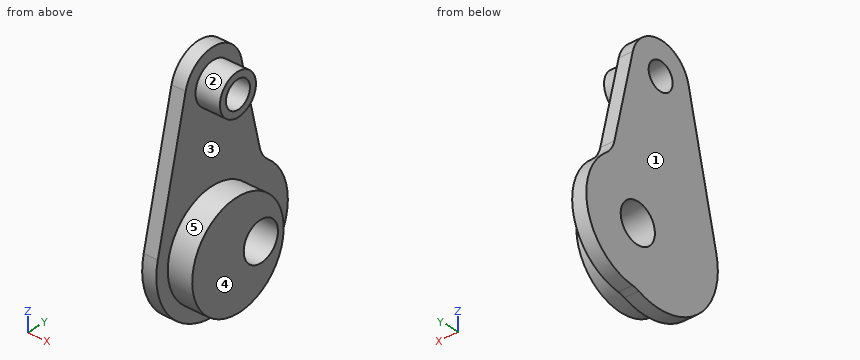
Autodesk Inventor part; units mm, degrees
ref_plane "YZ Plane" through (0, 0, 0) normal (1, 0, 0) x (0, 1, 0)
ref_plane "XZ Plane" through (0, 0, 0) normal (0, 1, 0) x (-1, 0, 0)
ref_plane "XY Plane" through (0, 0, 0) normal (0, 0, 1) x (1, 0, 0)
sketch "スケッチ1" plane through (0, 0, 0) normal (1, 0, 0) x (0, 1, 0)
  line L0 (0, 0) -> (0, -11) construction
  arc A0 (2.4346, 0.5682) -> (-2.4346, 0.5682) centre (0, 0) ccw
  circle A1 centre (0, -11) radius 4 construction
  line L1 (-2.4346, 0.5682) -> (-4.8692, -9.8636)
  arc A2 (0, -2.5) -> (2.4346, 0.5682) centre (0, 0) ccw construction
  arc A3 (-2.4346, 0.5682) -> (0, -2.5) centre (0, 0) ccw construction
  arc A4 (-4.8692, -9.8636) -> (1.9196, -15.6168) centre (0, -11) ccw
  arc A5 (-0.8211, -15.9321) -> (2.1875, -15.4961) centre (0, -11) ccw construction
  line L2 (2.4346, 0.5682) -> (4.043, -6.3238)
  arc A6 (2.476, -15.4748) -> (4.7628, -7.448) centre (2, -11) ccw
  line L3 (0, -11) -> (2, -11) construction
  arc A7 (0, -6) -> (-4.8692, -9.8636) centre (0, -11) ccw construction
  arc A8 (4.043, -6.3238) -> (4.7628, -7.448) centre (5.9907, -5.8693) ccw
  arc A9 (2.476, -15.4748) -> (1.9196, -15.6168) centre (2.6875, -17.4635) ccw
  point P0 (4.221, -7.0863)
  dimension "d1" = 11
  dimension "d2" = 8
  dimension "d4" = 2.5
  dimension "d39" = 5
  dimension "d54" = 2
  dimension "d55" = 4.5
  dimension "d56" = 2
extrude "押し出し1" add sketch "スケッチ1" along normal blind 1.1
sketch "スケッチ2" plane through (1.1, 0, 0) normal (1, 0, 0) x (0, 0, -1)
  circle A0 centre (0, 0) radius 1.575
  circle A1 centre (11, 0) radius 4
  line L0 (0, 0) -> (11, 0) construction
  arc A2 (9.8636, -4.8692) -> (15.6168, 1.9196) centre (11, 0) ccw construction
  point P0 (8.75, 4.8412)
  dimension "d12" = 3.15
  dimension "d13" = 8
extrude "押し出し2" add sketch "スケッチ2" along normal blind 1.9
sketch "スケッチ3" plane through (1.1, 0, 0) normal (1, 0, 0) x (0, 0, -1)
  point P0 (0, 0)
sketch "スケッチ4" plane through (0, 0, 0) normal (-1, 0, 0) x (0, 0, 1)
  arc A0 (0.5682, -2.4346) -> (0.5682, 2.4346) centre (0, 0) ccw construction
  arc A1 (-15.6168, 1.9196) -> (-9.8636, -4.8692) centre (-11, 0) ccw construction
  line L0 (-11, 0) -> (-11, 2) construction
  dimension "d53" = 2
hole "穴3" at (0, 0, 0) direction (1, 0, 0) diameter 2.1 end through all
hole "穴4" at (0, 2, -11) direction (1, 0, 0) diameter 2.99 end through all
properties part number "UPPER_LEG_BELT_TENSIONER"
Could you check a few things on this model? Use its own coordinates, in mm. Face numbers are marked on the shaded views. A direction names the side the tool comes from. Coordinates: 2 decimals unless noted, no trailing zeros. Order: outer loops, then holes, each group sorted by start corner. A loop starts at its lowest first (then second) coordinate and runs counter-clockwise, first axis right, second up. Notation, with made-up numbers: (-8.5, 35.5) -> (28.5, 35.5) arc R23 ccw to (28.5, 55.5) -> close; hole circle Ø5 at (78, -14.75). An arc over 180 degrees is marked (long way). One line per item, written item: value. Start each with the question number.
1) Imagine slicing it at D-D on x = 0.55. List the corners of the cut face in (y, z) for me (3 decimals), plus the area to 3 significant figures.
2) We'd pull the mould along Z, two halves only. Please class the marked faces 1, 2 and 3: +Z half, -Z half, draft (parallel to the pull), parting line (faces both ways), or undercut.
3) Imagine slicing it at C-C on x = 1.7. List the corners of the cut face in (y, z) for me (3 decimals).
4) Imagine slicing it at B-B on y = 0. List the corners of the cut face in (x, z) for me (3 decimals).
5) Imagine slicing it at A-A on z = -11. List the corners of the cut face in (x, y) for me (3 decimals), plus the area to 3 significant figures.
6) I'm going to push a flat-ended pin straight in: pin 1 (5 mm diameter, centred on y = 2, z = -11, fed in from -X). Where does the tip first touch, or does it pass through?
7) If I drill on L1, parallel to Y at x = 1.8, z = 0 (3 decimals); L2, parallel to Y at x = 1.5, z = -11 (3 decimals); L3, parallel to Z at x = 1.55, y = -0.25, over which ranges is the centre line in solid material (lowest first)? Write a range as [from, to].
8) Which directions (+Z, -Z, +X, -X, +Y, -Y) give clear straight access to the entire face, cutting with the end or side of a thin tool? Please do the marked faces 4 and 5.
Answer list:
1. outline: (-4.869, -9.864) arc R5 ccw to (1.92, -15.617) arc R2.004 cw to (2.476, -15.475) arc R4.5 ccw to (4.763, -7.448) arc R2 cw to (4.043, -6.324) -> (2.435, 0.568) arc R2.5 ccw to (-2.435, 0.568) -> close; hole circle Ø2.1 at (0, 0); hole circle Ø2.99 at (2, -11)
1. area: 134 mm2
2. face 1: draft
2. face 2: undercut
2. face 3: undercut
3. outline: circle Ø8 at (0, -11); circle Ø3.15 at (0, 0); hole circle Ø2.1 at (0, 0); hole circle Ø2.99 at (2, -11)
4. outline: (0, -16) -> (1.1, -16) -> (1.1, -15) -> (3, -15) -> (3, -7) -> (1.1, -7) -> (1.1, -1.575) -> (3, -1.575) -> (3, -1.05) -> (0, -1.05) -> close; (0, 1.05) -> (3, 1.05) -> (3, 1.575) -> (1.1, 1.575) -> (1.1, 2.5) -> (0, 2.5) -> close
5. outline: (0, -5) -> (1.1, -5) -> (1.1, -4) -> (3, -4) -> (3, 0.505) -> (0, 0.505) -> close; (0, 3.495) -> (3, 3.495) -> (3, 4) -> (1.1, 4) -> (1.1, 6.5) -> (0, 6.5) -> close
5. area: 18.9 mm2
6. pin 1: stops at x = 0
7. L1: y = [-1.575, -1.05], [1.05, 1.575]
7. L2: y = [-4, 0.505], [3.495, 4]
7. L3: z = [-14.99, -7.01], [-1.56, -1.02], [1.02, 1.56]
8. face 4: +Z, -Z, +X, +Y, -Y
8. face 5: +X
